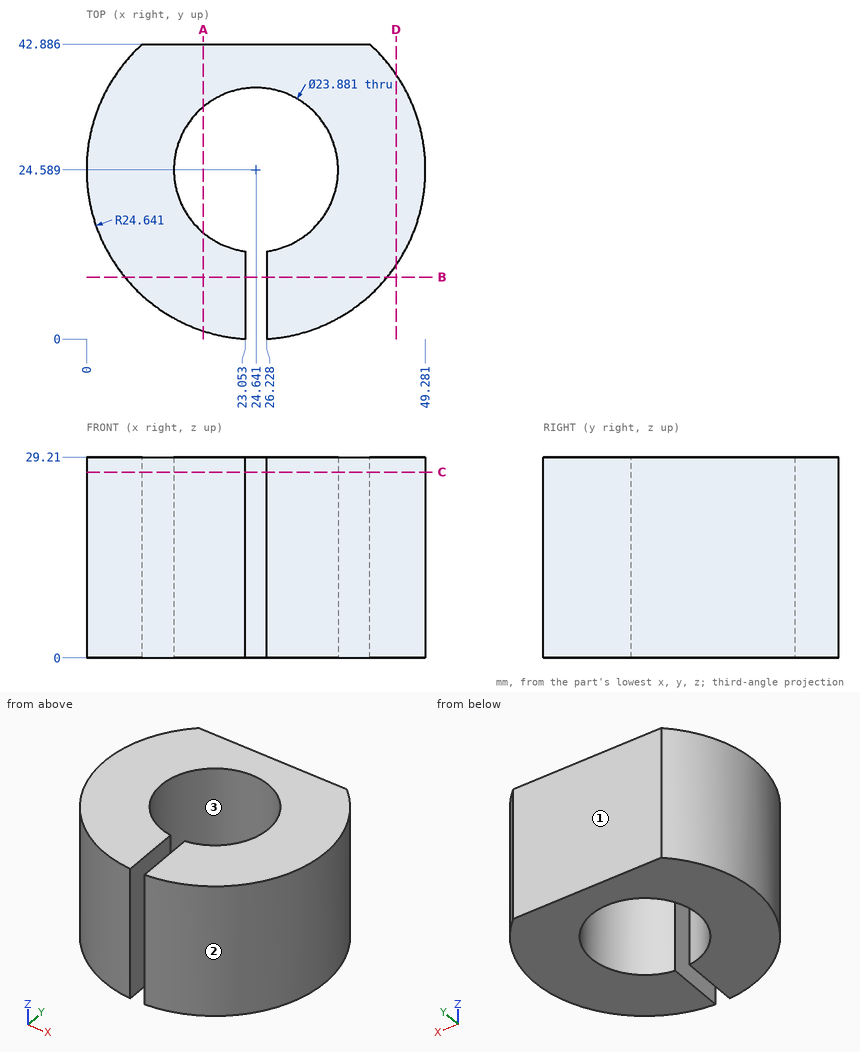
Verification items for this drawing (mm, ordinates from the low corner). Coordinates: 2 decimals unless noted, no trailing zeros. Loops run counter-clockwise (first coordinate to the right, second up) from the corner with the lowest first, then second, coordinate; pieces in that order, holes last.
Item 1: Release check for a two-part mould opening along Y. For the marked faces 1, 2 and 3 record: released by +Y, released by -Y, zero draft, split by the parting line, or undercut.
Item 2: Sectioned sample at A-A, the plane x = 17. Record the boundary of the cut face in (y, z) (1 decimal).
Item 3: Go/stop test with flat-tipped pins: pin 1 Ø5 at (y, z) = (7.5, 11) entering from +X; pin 2 Ø14 at (y, z) = (6.5, 11.5) entering from -X; pin 3 Ø3 at (y, z) = (28, 5.5) entering from +X; pin 4 Ø8 at (x, y) = (29, 25.5) entering from +Z. Record where each tip stops, or that it passes through.
Item 4: Thickness scan on line 1 (X direction, y = 25, z = 16.25) (1 decimal); line 2 (Y direction, x = 15, z = 15.25) (1 decimal); line 3 (X direction, y = 16, z = 4.25) (1 decimal). Record the ranges inside material, lowest first.
Item 5: Sectioned sample at B-B, the plane y = 9. Record the boundary of the cut face in (x, z), then the cut area to 3 significant figures.
Item 6: Sectioned sample at C-C, the plane z = 27. Record the boundary of the cut face in (x, y) (1 decimal), then the cut area to 3 significant figures.
Item 7: Sectioned sample at D-D, the plane x = 45. Record the boundary of the cut face in (y, z), then the cut area to 3 significant figures.
Check result:
1. face 1: released by +Y
1. face 2: split by the parting line
1. face 3: undercut
2. outline: (1.2, 0) - (15.4, 0) - (15.4, 29.2) - (1.2, 29.2) - close; (33.8, 0) - (42.9, 0) - (42.9, 29.2) - (33.8, 29.2) - close
3. pin 1: stops at x = 44.5
3. pin 2: stops at x = 2.64
3. pin 3: stops at x = 49.21
3. pin 4: passes through
4. line 1: x = 0 to 12.7, 36.6 to 49.3
4. line 2: y = 1.9 to 17.5, 31.6 to 42.9
4. line 3: x = 1.5 to 16.3, 32.9 to 47.7
5. outline: (5.56, 0) - (23.05, 0) - (23.05, 29.21) - (5.56, 29.21) - close; (26.23, 0) - (43.72, 0) - (43.72, 29.21) - (26.23, 29.21) - close
5. area: 1,020 mm2
6. outline: (8.1, 42.9) arc R24.6 ccw to (23.1, 0) - (23.1, 12.8) arc R11.9 cw (long way) to (26.2, 12.8) - (26.2, 0) arc R24.6 ccw to (41.1, 42.9) - close
6. area: 1,280 mm2
7. outline: (10.71, 0) - (38.47, 0) - (38.47, 29.21) - (10.71, 29.21) - close
7. area: 811 mm2
